Input: part model. Units: mm. Frame: model coordinates. A direction names the side the tool comes from. Give positions to 0.01 mm unless a question says otherwise; leave off trailing zeros. Write each loop counter-clockwise with the first axis right and the second up, starting at its lowest first coordinate (ties: lowest second). Pieces come first, ordered by that corner, then holes.
Autodesk Inventor part; units mm, degrees
ref_plane "РабПлоскость8" through (0, -13.3, 0) normal (1, 0, 0) x (0, 0, -1)
ref_plane "YZ Plane" through (0, 0, 0) normal (1, 0, 0) x (0, 1, 0)
ref_plane "XZ Plane" through (0, 0, 0) normal (0, 1, 0) x (-1, 0, 0)
sketch "Эскиз1" plane through (0, 0, 0) normal (0, 0, 1) x (1, 0, 0)
  circle A0 centre (0, 0) radius 5.75
  circle A1 centre (0, 0) radius 9.55
  line L0 (9.55, 13.5) -> (-9.55, 13.5)
  line L1 (-9.55, 13.5) -> (-9.55, 0)
  line L2 (-9.55, 0) -> (9.55, 0)
  line L3 (9.55, 0) -> (9.55, 13.5)
  line L4 (9.55, 0) -> (-9.55, 0)
  line L5 (-9.55, 0) -> (-9.55, -13.3)
  line L6 (-9.55, -13.3) -> (9.55, -13.3)
  line L7 (9.55, -13.3) -> (9.55, 0)
  point P0 (9.55, 0)
  point P1 (0, 9.55)
  point P2 (-9.55, 0)
  point P3 (9.55, 0)
  point P4 (-9.55, 0)
  point P5 (-4.7236, -8.3)
  point P6 (4.7236, -8.3)
  point P7 (-9.55, 0)
  point P8 (9.55, 0)
  dimension "d0" = 11.5
  dimension "d1" = 19.1
  dimension "d64" = 13.3
  dimension "d85" = 13.5
extrude "Выдавливание1" add sketch "Эскиз1" along normal blind 8 contours L2 A1 A0 | A0 L2 A1 | L7 L6 L5 A1 | A1 L1 L0 L3
ref_plane "РабПлоскость8" through (0, -13.3, 0) normal (1, 0, 0) x (0, 0, -1)
sketch "Эскиз15" plane through (0, 0, 8) normal (0, 0, 1) x (1, 0, 0)
  circle A0 centre (0, 0) radius 5.75
  circle A1 centre (0, 0) radius 7.55
  dimension "d67" = 15.1
extrude "Выдавливание9" cut sketch "Эскиз15" against normal blind 4
sketch "Эскиз16" plane through (-9.55, -13.3, 0) normal (0, -1, 0) x (1, 0, 0)
  line L0 (0, 8) -> (19.1, 8)
  line L1 (19.1, 8) -> (24.7, 8)
  line L2 (24.7, 8) -> (24.7, 0)
  line L3 (24.7, 0) -> (19.1, 0)
  line L4 (19.1, 0) -> (19.1, 8)
  point P0 (9.55, 0)
  dimension "d70" = 5.6
  dimension "d71" = 8
extrude "Выдавливание10" add sketch "Эскиз16" against normal up to surface (26.8 mm away)
sketch "Эскиз17" plane through (-9.55, 13.5, 0) normal (0, 1, 0) x (1, 0, 0)
  line L0 (24.7, 0) -> (24.7, -8)
  line L1 (24.7, -4) -> (20.15, -4)
  point P0 (9.55, 0)
  dimension "d82" = 4.55
hole "Отверстие4" at (10.6, 13.5, 4) direction (0, -1, 0) diameter 3.2 end through all
fillet "Сопряжение5" radius 2.95 1 edges at (15.15, 0.1, 0)
mirror "Зеркальное отражение5" about plane through (0, -13.3, 0) normal (1, 0, 0) of "Сопряжение5", "Отверстие4", "Выдавливание10", "Выдавливание9"
fillet "Сопряжение6" radius 5.05 1 edges at (15.15, 0.1, 8)
sketch "Эскиз18" plane through (0, 0, 8) normal (0, 0, 1) x (1, 0, 0)
  circle A0 centre (0, 0) radius 7.55
  circle A1 centre (0, 16.1) radius 7.55
  circle A2 centre (0, -16.1) radius 7.55
  dimension "d86" = 16.1
  dimension "d90" = 16.1
extrude "Выдавливание11" cut sketch "Эскиз18" against normal through all contours A1 | A2
properties part number "Крепление дифференциала"
Q1. Mould query, pull axis Z, two halves, no side actions, for faces 3 (the cylindrical face through (-0.13, 8.55, 4.06)), 4 (the cylindrical face through (12.16, -0.09, 3.65)), 5 (the flat face through (0, 6, 0)), 6 (the cylindrical face through (13.63, 0.29, 6.56)). Classes: +Z half, -Z half, draft (parallel to the pull), parting line (faces both ways), or undercut.
Q2. Section A-A, the plane y = -11.5. Give the number of separate pieces and of enclosed holes in the cut face, then the cut area to 3 significant figures.
Q3. Section B-B, the plane x = 0. Return the cut outline in (y, z).
Q4. Section C-C, the plane z = 7.5. Return the cut outline in (x, y).
Q5. Material intervals for line 1 along Z through (x, y) = (-10.6, -6.5); line 2 along X through (y, z) = (3, 5); line 3 along X through (y, z) = (0, 2.8), sorted ascending.
Q6. Access query for faces 1 (the flat face through (-2, -6, 4)), 2 (the cylindrical face through (0.13, -8.55, 4.06)). Directions: +Z, -Z, +X, -X, +Y, -Y. A direction counts if a zero-diameter tool reaches every point of the face in a straight line with its end or side. Return the directions, or none.
Q7. Pin query (flat end, axial travel): pin 1 (3 mm diameter, centred on x = 2, z = 6.5, fed in from +Y); pin 2 (13 mm diameter, centred on x = 0, y = 0, fed in from +Z); pin 3 (2 mm diameter, centred on y = -1.5, z = 1, fed in from -X); pin 4 (1.9 mm diameter, centred on x = 10.6, z = 4, fed in from +Y). Return the tip coordinate at first contact, or that it passes through.
Solutions:
1. face 3: draft
1. face 4: undercut
1. face 5: -Z half
1. face 6: +Z half
2. separate pieces: 2
2. enclosed holes: 2
2. area: 121 mm2
3. outline: (-8.55, 0) - (-5.75, 0) - (-5.75, 4) - (-7.55, 4) - (-7.55, 8) - (-8.55, 8) - close; (5.75, 0) - (8.55, 0) - (8.55, 8) - (7.55, 8) - (7.55, 4) - (5.75, 4) - close
4. outline: (-15.15, -13.3) - (-7.01, -13.3) arc R7.55 cw to (7.01, -13.3) - (12.29, -13.3) - (12.29, 13.5) - (7.09, 13.5) arc R7.55 cw to (-7.09, 13.5) - (-15.15, 13.5) - close; hole circle Ø15.1 at (0, 0)
5. line 1: z = 0 to 2.4, 5.6 to 8
5. line 2: x = -15.15 to -11.85, -9.35 to -6.93, 6.93 to 9.35, 11.85 to 14.72
5. line 3: x = -15.15 to -11.66, -9.54 to -5.75, 5.75 to 9.54, 11.66 to 15.15
6. face 1: +Z
6. face 2: +Z, -Z, -Y
7. pin 1: stops at y = 9.41
7. pin 2: stops at z = 4
7. pin 3: stops at x = -14.99
7. pin 4: passes through
